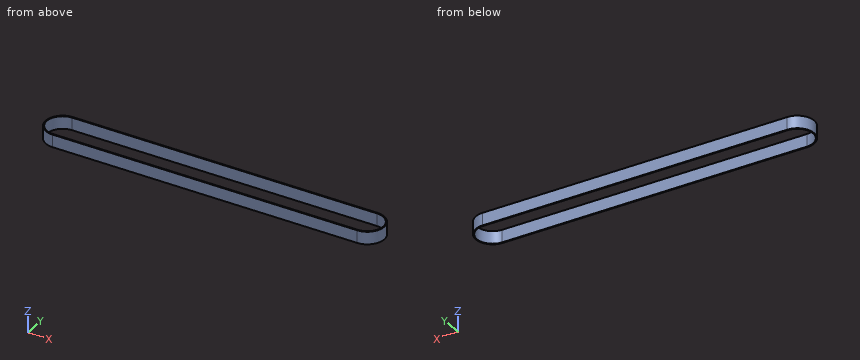
from build123d import *

# Parameters (mm, degrees)
EXTRUDE_THIN1_START = -0.5
EXTRUDE_THIN1_DEPTH = 6


with BuildPart() as part:
    # Sketch2 → Extrude-Thin1 (new body)
    with BuildSketch(Plane.XY.offset(EXTRUDE_THIN1_START)):
        with BuildLine():
            Line((145, -8.5), (0, -8.5))
            ThreePointArc((0, -8.5), (-8, -0.5), (0, 7.5))
            Line((0, 7.5), (145, 7.5))
            ThreePointArc((145, 7.5), (153, -0.5), (145, -8.5))
        make_face()
        with BuildLine():
            Line((145, -8), (0, -8))
            ThreePointArc((0, -8), (-7.5, -0.5), (0, 7))
            Line((0, 7), (145, 7))
            ThreePointArc((145, 7), (152.5, -0.5), (145, -8))
        make_face(mode=Mode.SUBTRACT)
    extrude(amount=-EXTRUDE_THIN1_DEPTH)


solid = part.part
The listing builds one solid part. Answer for the finished solid, in the listing's coordinates (mm). Coordinates: 2 decimals unless noted, no trailing zeros. Loops run counter-clockwise (first coordinate to the right, second up) from the corner with the lowest first, then second, coordinate; pieces in that order, holes last. Notation, with made-up numbers: (71, 43.5) -> (98, 43.5) arc R26 cw to (98, 59.5) -> close; hole circle Ø9 at (78.25, -39). An arc over 180 degrees is marked (long way). Answer in a Markdown table with one row per item. Add a question column.
1. The part is cut by section A-A, the plane y = -0.5. Write down the section's boundary in (x, z).
2. The part is cut by section B-B, the plane x = 67.5. Write down the section's boundary in (y, z), then the cut area to 3 significant figures.
3. The part is cut by section C-C, the plane z = -2.2. Write down the section's boundary in (x, y), then the cut area to 3 significant figures.
4. Flat-ended cylindrical pins translate along their axes: P1, Ø8, axis at x = 16, y = -1.5, coming from the -Z side; P2, Ø3, axis at y = 3, z = -4, coming from the +X side; P3, Ø3, axis at y = -5.5, z = -1.5, coming from the -X side. Find the tip coordinate at first contact, or state that the pin passes through.
5. Consider line 1 (X direction, y = -0.75, z = -4.1); line 2 (Y direction, x = 31, z = -3.55); line 3 (X direction, y = -7, z = -5.4). Determine where each line is inside the solid, lowest interval first. Write a range as [from, to].
Answer below:
| question | item | result |
|---|---|---|
| 1 | outline | (-8, -6.5) -> (-7.5, -6.5) -> (-7.5, -0.5) -> (-8, -0.5) -> close; (152.5, -6.5) -> (153, -6.5) -> (153, -0.5) -> (152.5, -0.5) -> close |
| 2 | outline | (-8.5, -6.5) -> (-8, -6.5) -> (-8, -0.5) -> (-8.5, -0.5) -> close; (7, -6.5) -> (7.5, -6.5) -> (7.5, -0.5) -> (7, -0.5) -> close |
| 2 | area | 6.00 mm2 |
| 3 | outline | (0, -8.5) -> (145, -8.5) arc R8 ccw to (145, 7.5) -> (0, 7.5) arc R8 ccw to start; hole (0, -8) -> (145, -8) arc R7.5 ccw to (145, 7) -> (0, 7) arc R7.5 ccw to start |
| 3 | area | 169 mm2 |
| 4 | P1 | through |
| 4 | P2 | x = 152.75 |
| 4 | P3 | x = -7.19 |
| 5 | line 1 | [-8, -7.5], [152.5, 153] |
| 5 | line 2 | [-8.5, -8], [7, 7.5] |
| 5 | line 3 | [-4.66, -3.74], [148.74, 149.66] |
